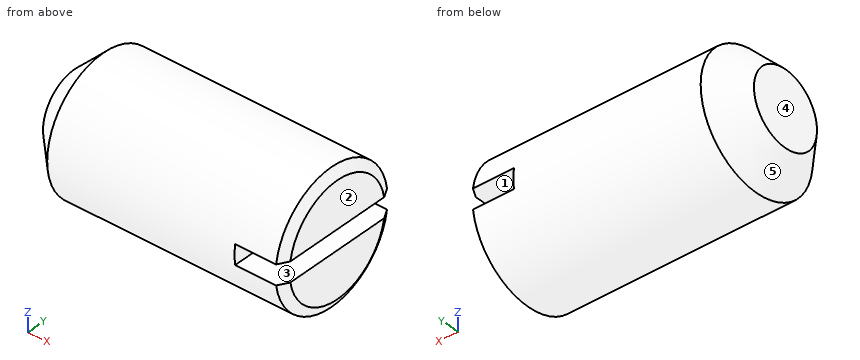
from build123d import *

# Parameters (mm, degrees)
SKICA2_W                 = 0.6
SKICA2_H                 = 4
ODEBRAT_VYSUNUT_M1_DEPTH = 1.42


with BuildPart() as part:
    # Skica1 → Otočit kolem osy1 (revolve)
    with BuildSketch(Plane(origin=(0, 0, 0), x_dir=(1, 0, 0), z_dir=(0, 1, 0))):
        Polygon((0, 0), (0, 1.125), (0.875, 2), (7.826794919, 2), (8, 1.7), (8, 0), align=None)
    revolve(axis=Axis((8, 0, 0), (-1, 0, 0)))

    # Skica2 → Odebrat vysunutím1 (cut)
    with BuildSketch(Plane(origin=(8, 0, 0), x_dir=(0, 0, -1), z_dir=(1, 0, 0))):
        Rectangle(SKICA2_W, SKICA2_H)
    extrude(amount=-ODEBRAT_VYSUNUT_M1_DEPTH, mode=Mode.SUBTRACT)


solid = part.part
CAD build for the part. Positions are in the model's coordinates, mm. Face numbers are marked on the shaded views. A direction names the side the tool comes from. Round coordinates to 2 decimals unless told otherwise and drop trailing zeros. Order: outer loops, then holes, each group sorted by start corner. A loop starts at its lowest first (then second) coordinate and runs counter-clockwise, first axis right, second up. Notation, with made-up numbers: M 17.25,-34.75 L 23.25,-34.75 A15 ccw 23.25,-7.75 Z; hole C 87.25,41.5 d9. An arc over 180 degrees is marked long. Use one line per item in the form item = value.
Q1. Which spindle directions (+Z, -Z, +X, -X, +Y, -Y) get a long thin tool onto all of the face, cutting with end or side? Do the marked faces 1 and 2. Say none if no direction does.
Recorded:
face_1 = +X, +Y, -Y
face_2 = +Z, -Z, +X, +Y, -Y
Q2. Probe L1, parallel to Z at x = 6.75, y = -1.1; L2, parallel to Z at x = 7.25, y = -1.4; L3, parallel to X at y = -0.5, z = -0.05. List the from-to ranges inside material, lowest first.
Recorded:
L1 = -1.67 to -0.3, 0.3 to 1.67
L2 = -1.43 to -0.3, 0.3 to 1.43
L3 = 0 to 6.58
Q3. Flat gauge pins, fed straight in: P1, Ø2, axis at x = 6, y = 0.5, coming from the +Z side; P2, Ø1.5, axis at x = 6, z = -1.5, coming from the +Y side. Where does each tip first touch, or does it go through?
Recorded:
P1 = 2
P2 = 1.85
Q4. Saw through at B-B on y = 0. Give the cut face in (x, z) (3 decimals), then the cut area to 3 significant figures.
Recorded:
outline = M 0,-1.125 L 0.875,-2 L 7.827,-2 L 8,-1.7 L 8,-0.3 L 6.58,-0.3 L 6.58,0.3 L 8,0.3 L 8,1.7 L 7.827,2 L 0.875,2 L 0,1.125 Z
area = 30.3 mm^2
Q5. Two-plate mould, pull along Z, no slides. Class the marked faces 3, 4 and 5: +Z half, -Z half, draft (parallel to the pull), parting line (faces both ways), or undercut.
Recorded:
face_3 = undercut
face_4 = draft
face_5 = parting line
Q6. Saw through at A-A on x = 6.75. Give the cut face in (y, z), then the cut area to 3 significant figures.
Recorded:
outline = M -1.98,-0.3 A2 ccw 1.98,-0.3 Z; M -1.98,0.3 L 1.98,0.3 A2 ccw Z
area = 10.2 mm^2
Q7. Saw through at C-C on z = 0. Give the cut face in (x, y) (3 decimals), then the cut area to 3 significant figures.
Recorded:
outline = M 0,-1.125 L 0.875,-2 L 6.58,-2 L 6.58,2 L 0.875,2 L 0,1.125 Z
area = 25.6 mm^2
